from build123d import *

# Parameters (mm, degrees)
F0_W     = 47
F0_H     = 50
F0_R     = 1.5
F1_DEPTH = 5


# Not quite as in the source:
# - a feature names something its author has since deleted; it is built from what else it names


with BuildPart() as f1:
    # F0 (on Front) → F1 (new body)
    with BuildSketch(Plane.XZ):
        with Locations((23.5, 25)):
            Rectangle(F0_W, F0_H)
        with BuildLine():
            ThreePointArc((9.5, 11), (6.6141807012, 10.4259748515), (9.0606601718, 12.0606601718))
            ThreePointArc((9.0606601718, 12.0606601718), (9.3858192988, 11.5740251485), (9.5, 11))
        make_face(mode=Mode.SUBTRACT)
        with Locations((39, 11)):
            Circle(F0_R, mode=Mode.SUBTRACT)
        with BuildLine():
            ThreePointArc((14.6611652352, 17.6611652352), (14.6611652352, 35.3388347648), (32.3388347648, 35.3388347648))
            ThreePointArc((32.3388347648, 35.3388347648), (35.0484941564, 31.2835429046), (36, 26.5))
            ThreePointArc((36, 26.5), (28.2835429046, 14.9515058436), (14.6611652352, 17.6611652352))
        make_face(mode=Mode.SUBTRACT)
        with Locations((8, 42)):
            Circle(F0_R, mode=Mode.SUBTRACT)
        with BuildLine():
            ThreePointArc((37.9393398282, 40.9393398282), (38.4259748515, 43.3858192988), (40.5, 42))
            ThreePointArc((40.5, 42), (39.5740251485, 40.6141807012), (37.9393398282, 40.9393398282))
        make_face(mode=Mode.SUBTRACT)
        with BuildLine():
            Line((47, 50), (47, 0))
            Line((47, 0), (47, -12.5))
            Line((47, -12.5), (51.5, -12.5))
            ThreePointArc((51.5, -12.5), (53.5, -10.5), (55.5, -12.5))
            Line((55.5, -12.5), (65.5, -12.5))
            Line((65.5, -12.5), (65.5, 26.5))
            Line((65.5, 26.5), (65.5, 50))
            Line((65.5, 50), (61.5, 50))
            Line((61.5, 50), (47, 50))
        make_face()
        with BuildLine():
            ThreePointArc((56, 17.5), (51.732233047, 15.732233047), (53.5, 20))
            ThreePointArc((53.5, 20), (55.267766953, 19.267766953), (56, 17.5))
        make_face(mode=Mode.SUBTRACT)
        with BuildLine():
            ThreePointArc((53.5, 22.5), (50.6715728753, 29.3284271247), (57.5, 26.5))
            ThreePointArc((57.5, 26.5), (56.3284271247, 23.6715728753), (53.5, 22.5))
        make_face(mode=Mode.SUBTRACT)
        with BuildLine():
            ThreePointArc((63, 38), (60.4393398282, 36.9393398282), (61.5, 39.5))
            ThreePointArc((61.5, 39.5), (62.5606601718, 39.0606601718), (63, 38))
        make_face(mode=Mode.SUBTRACT)
        with BuildLine():
            ThreePointArc((61.5, 43.5), (60, 45), (61.5, 46.5))
            ThreePointArc((61.5, 46.5), (62.5606601718, 46.0606601718), (63, 45))
            ThreePointArc((63, 45), (62.5606601718, 43.9393398282), (61.5, 43.5))
        make_face(mode=Mode.SUBTRACT)
        with BuildLine():
            Line((47, 0), (0, 0))
            Line((0, 0), (0, -12.5))
            Line((0, -12.5), (10, -12.5))
            ThreePointArc((10, -12.5), (12, -10.5), (14, -12.5))
            Line((14, -12.5), (30, -12.5))
            ThreePointArc((30, -12.5), (32, -10.5), (34, -12.5))
            Line((34, -12.5), (47, -12.5))
            Line((47, -12.5), (47, 0))
        make_face()
        with BuildLine():
            Line((10, -12.5), (0, -12.5))
            Line((0, -12.5), (0, -25))
            Line((0, -25), (47, -25))
            Line((47, -25), (47, -12.5))
            Line((47, -12.5), (34, -12.5))
            ThreePointArc((34, -12.5), (32, -14.5), (30, -12.5))
            Line((30, -12.5), (14, -12.5))
            ThreePointArc((14, -12.5), (12, -14.5), (10, -12.5))
        make_face()
        with BuildLine():
            Line((51.5, -12.5), (47, -12.5))
            Line((47, -12.5), (47, -25))
            Line((47, -25), (65.5, -25))
            Line((65.5, -25), (65.5, -12.5))
            Line((65.5, -12.5), (55.5, -12.5))
            ThreePointArc((55.5, -12.5), (53.5, -14.5), (51.5, -12.5))
        make_face()
    extrude(amount=F1_DEPTH)


solid = f1.part
Here's how the part is built. I have some questions about the finished solid (model axes, mm). Round coordinates to 2 decimals unless told otherwise and drop trailing zeros. Order: outer loops, then holes, each group sorted by start corner. A loop starts at its lowest first (then second) coordinate and runs counter-clockwise, first axis right, second up. Notation, with made-up numbers: (39.5, 71.25) -> (77.5, 71.25) arc R17 cw to (77.5, 79.25) -> close; hole circle Ø8 at (40.5, 55.25). An arc over 180 degrees is marked (long way). Return JSON: item names as keys, results as strings.
Q1. For pin 1 Ø6.5 at (x, z) = (12, -12.5) entering from +Y; pin 2 Ø2.5 at (x, z) = (8, 11) entering from +Y, each with a flat end and sliding along its axis, tell me the tip position at first contact or that it passes through.
Filled sheet:
{"pin 1": "stops at y = 0", "pin 2": "passes through"}
Q2. If we section it at A-A on x = 39: List the corners of the cut face in (y, z) for me, plus the area to 3 significant figures.
Filled sheet:
{"outline": "(-5, -25) -> (0, -25) -> (0, 9.5) -> (-5, 9.5) -> close; (-5, 12.5) -> (0, 12.5) -> (0, 40.5) -> (-5, 40.5) -> close; (-5, 43.5) -> (0, 43.5) -> (0, 50) -> (-5, 50) -> close", "area": "345 mm^2"}
Q3. If we mould it in two halves opening along X, with no side actions, what happens to faces 1 (the flat face through (32, -5, 13)), 2 (the cylindrical face through (7.675, -2.465, 40.536)), 3 (the flat face through (0, -2, 13))? For each: released by +X, released by -X, zero draft, split by the parting line, or undercut.
Filled sheet:
{"face 1": "zero draft", "face 2": "undercut", "face 3": "released by -X"}
Q4. If we section it at D-D on x = 23.5: List the corners of the cut face in (y, z) for me, plus the area to 3 significant figures.
Filled sheet:
{"outline": "(-5, -25) -> (0, -25) -> (0, 14) -> (-5, 14) -> close; (-5, 39) -> (0, 39) -> (0, 50) -> (-5, 50) -> close", "area": "250 mm^2"}
Q5. If we section it at C-C on y = -1.05: Give the number of separate pieces and of enclosed holes in the cut face, plus the area to 3 significant figures.
Filled sheet:
{"separate pieces": "1", "enclosed holes": "12", "area": "4,270 mm^2"}
Q6. I need wall thicknesses on line 1 along Z through (x, y) = (53.5, -1.2); line 2 along Z through (x, y) = (39, -2); line 3 along X through (y, z) = (-3.2, -12.5). Which ranges of each line are inside material? Lowest first, please. Write a range as from..to.
Filled sheet:
{"line 1": "z = -25..-14.5, -10.5..15, 20..22.5, 30.5..50", "line 2": "z = -25..9.5, 12.5..40.5, 43.5..50", "line 3": "x = 0..10, 14..30, 34..51.5, 55.5..65.5"}
Q7. If we section it at B-B on z = -12.5: List the corners of the cut face in (x, y) for me.
Filled sheet:
{"outline": "(0, -5) -> (10, -5) -> (10, 0) -> (0, 0) -> close; (14, -5) -> (30, -5) -> (30, 0) -> (14, 0) -> close; (34, -5) -> (51.5, -5) -> (51.5, 0) -> (34, 0) -> close; (55.5, -5) -> (65.5, -5) -> (65.5, 0) -> (55.5, 0) -> close"}
